Here's how the part is built. I have some questions about the finished solid (model axes, mm). Coordinates: 2 decimals unless noted, no trailing zeros. Write each loop counter-clockwise with the first axis right and the second up, starting at its lowest first coordinate (ties: lowest second). Pieces come first, ordered by that corner, then holes. Notation, with made-up numbers: M 43,35 L 87,35 A24 ccw 87,53 Z; hole C -33.75,55 d9. An arc over 180 degrees is marked long. Use one line per item in the form item = value. Start each with the question number.
1. I'm going to push flat-ended pins straight in: pin 1 Ø6.5 at (x, z) = (226, -5) entering from -Y; pin 2 Ø5 at (x, y) = (84.14, 45.21) entering from -Z; pin 3 Ø3 at (x, z) = (295.5, -9.5) entering from -Y. Where does each tip first touch, or does it pass through?
2. I want a section at B-B, the plane x = 186. List the corners of the cut face in (y, z) for me.
3. Thinking about a two-plate mould opening in X: for faces 1 (the face through (284.862, 34.561, -6.261)), 2 (the face through (288, 541, -12.7)), which applies, released by +X, released by -X, zero draft, split by the parting line, or undercut?
4. Please list where these lines run through material, in increasing order: line 1 along Y through (x, z) = (172, -8.75); line 2 along X through (y, z) = (91, -1.75); line 3 along Y through (x, z) = (283, -4). Write a range as [from, to].
5. I want a section at A-A, the plane z = -4.5. List the corners of the cut face in (x, y) for me, plus the area to 3 significant figures.
from build123d import *

# Parameters (mm, degrees)
PLAYFIELD_BLANK_W         = 584.2
PLAYFIELD_BLANK_H         = 1066.8
PLAYFIELD_THICKNESS_DEPTH = 12.7
SKETCH3_R                 = 3.1115
CUT_EXTRUDE1_DEPTH        = 12.7
CUT_EXTRUDE2_DEPTH        = 12.7
CUT_EXTRUDE3_DEPTH        = 12.7
CUT_EXTRUDE4_DEPTH        = 12.7


with BuildPart() as part:
    # Playfield_Blank → Playfield_Thickness (new body)
    with BuildSketch(Plane.XY):
        with Locations((292.1, 533.4)):
            Rectangle(PLAYFIELD_BLANK_W, PLAYFIELD_BLANK_H)
    extrude(amount=-PLAYFIELD_THICKNESS_DEPTH)

    # Sketch3 → Cut-Extrude1 (cut)
    with BuildSketch(Plane.XY):
        with Locations((84.136105728, 19.812)):
            Circle(SKETCH3_R)
        with Locations((84.136105728, 45.212)):
            Circle(SKETCH3_R)
        with Locations((88.898605728, 80.137)):
            Circle(SKETCH3_R)
        with Locations((485.773605728, 19.812)):
            Circle(SKETCH3_R)
        with Locations((485.773605728, 45.212)):
            Circle(SKETCH3_R)
        with Locations((478.788605728, 80.137)):
            Circle(SKETCH3_R)
    extrude(amount=-CUT_EXTRUDE1_DEPTH, mode=Mode.SUBTRACT)

    # Sketch4 → Cut-Extrude2 (cut)
    with BuildSketch(Plane.XY):
        with BuildLine():
            Line((0, 127), (31.75, 127))
            ThreePointArc((31.75, 127), (36.240128061, 125.140128061), (38.1, 120.65))
            Line((38.1, 120.65), (38.1, 0))
            Line((38.1, 0), (0, 0))
            Line((0, 0), (0, 127))
        make_face()
    extrude(amount=-CUT_EXTRUDE2_DEPTH, mode=Mode.SUBTRACT)

    # Sketch5 → Cut-Extrude3 (cut)
    with BuildSketch(Plane.XY):
        with BuildLine():
            Line((584.2, 105.791), (533.4, 105.791))
            ThreePointArc((533.4, 105.791), (527.05, 99.441), (533.4, 93.091))
            Line((533.4, 93.091), (533.4, 0))
            Line((533.4, 0), (584.2, 0))
            Line((584.2, 0), (584.2, 105.791))
        make_face()
    extrude(amount=-CUT_EXTRUDE3_DEPTH, mode=Mode.SUBTRACT)

    # Sketch7 → Cut-Extrude4 (cut)
    with BuildSketch(Plane.XY):
        with BuildLine():
            Line((158.326337108, 0), (158.326337108, 64.094614523))
            ThreePointArc((158.326337108, 64.094614523), (160.186209048, 68.584742584), (164.676337108, 70.444614523))
            Line((164.676337108, 70.444614523), (251.90120893, 70.444614523))
            ThreePointArc((251.90120893, 70.444614523), (254.5903795, 69.847080224), (256.773448763, 68.16693315))
            Line((256.773448763, 68.16693315), (313.748778564, 0))
            Line((313.748778564, 0), (158.326337108, 0))
        make_face()
    extrude(amount=-CUT_EXTRUDE4_DEPTH, mode=Mode.SUBTRACT)


solid = part.part
Answer list:
q1.pin_1 = 70.44
q1.pin_2 = through
q1.pin_3 = 20.04
q2.outline = M 70.44,-12.7 L 1066.8,-12.7 L 1066.8,0 L 70.44,0 Z
q3.face_1 = undercut
q3.face_2 = zero draft
q4.line_1 = [70.44, 1066.8]
q4.line_2 = [38.1, 533.4]
q4.line_3 = [36.79, 1066.8]
q5.outline = M 0,127 L 31.75,127 A6.35 cw 38.1,120.65 L 38.1,0 L 158.33,0 L 158.33,64.09 A6.35 cw 164.68,70.44 L 251.9,70.44 A6.35 cw 256.77,68.17 L 313.75,0 L 533.4,0 L 533.4,93.09 A6.35 cw 533.4,105.79 L 584.2,105.79 L 584.2,1066.8 L 0,1066.8 Z; hole C 84.14,19.81 d6.22; hole C 84.14,45.21 d6.22; hole C 88.9,80.14 d6.22; hole C 478.79,80.14 d6.22; hole C 485.77,19.81 d6.22; hole C 485.77,45.21 d6.22
q5.area = 604,000 mm²
